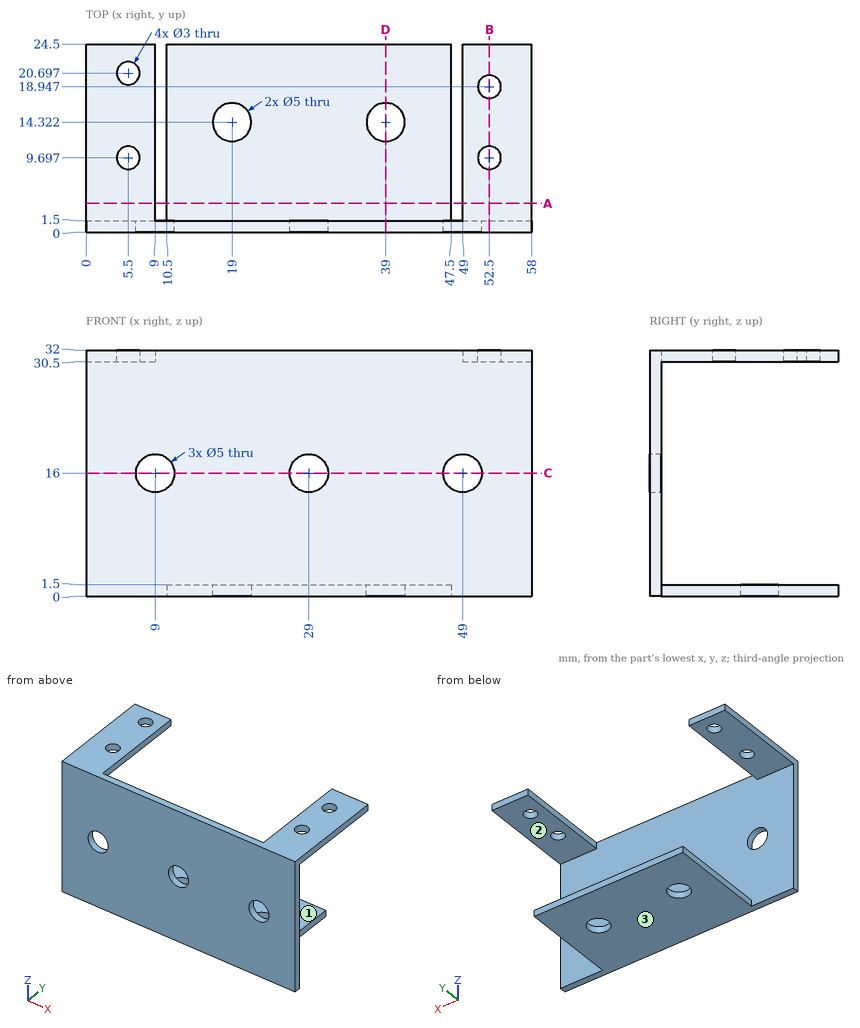
Job drawing, mm, ordinate dimensions from the low corner. One solid piece. A direction names the side the tool comes from. Coordinates: 2 decimals unless noted, no trailing zeros. Write each loop counter-clockwise with the first axis right and the second up, starting at its lowest first coordinate (ties: lowest second). Pieces come first, ordered by that corner, then holes.
Item 1: Which spindle directions (+Z, -Z, +X, -X, +Y, -Y) get a long thin tool onto all of the face, cutting with end or side? Do the marked faces 1, 2 and 3. Say none if no direction does.
Item 2: Slice it at B-B (x = 52.5). Write the cut outline in (y, z).
Item 3: Slice it at D-D (x = 39). Write the cut outline in (y, z).
Item 4: Slice it at C-C (z = 16). Write the cut outline in (x, y).
Item 5: Pin check, flat tips, straight feed: pin 1 (0.8 mm diameter, centred on y = 10.5, z = 0.5, fed in from +X); pin 2 (1.2 mm diameter, centred on y = 16, z = 0.5, fed in from -X); pin 3 (5 mm diameter, centred on x = 5.5, y = 9.7, fed in from -Z); pin 4 (4.5 mm diameter, centred on x = 29, z = 16, fed in from -Y). Stop position of each tip, or through.
Item 6: Probe line 1 (X direction, y = 0.85, z = 16); line 2 (Y direction, x = 52.5, z = 31.2); line 3 (Y direction, x = 5.5, z = 30.95). List the from-to ranges inside material, lowest first.
Item 7: Slice it at A-A (y = 3.75). Write the cut outline in (x, z).
Results found:
1. face 1: +Z, +X, -X, +Y
1. face 2: -Z, +X, -X, +Y
1. face 3: -Z, +X, -X, +Y, -Y
2. outline: (0, 0) - (1.5, 0) - (1.5, 30.5) - (8.2, 30.5) - (8.2, 32) - (0, 32) - close; (11.2, 30.5) - (17.45, 30.5) - (17.45, 32) - (11.2, 32) - close; (20.45, 30.5) - (24.5, 30.5) - (24.5, 32) - (20.45, 32) - close
3. outline: (0, 0) - (11.82, 0) - (11.82, 1.5) - (1.5, 1.5) - (1.5, 32) - (0, 32) - close; (16.82, 0) - (24.5, 0) - (24.5, 1.5) - (16.82, 1.5) - close
4. outline: (0, 0) - (6.5, 0) - (6.5, 1.5) - (0, 1.5) - close; (11.5, 0) - (26.5, 0) - (26.5, 1.5) - (11.5, 1.5) - close; (31.5, 0) - (46.5, 0) - (46.5, 1.5) - (31.5, 1.5) - close; (51.5, 0) - (58, 0) - (58, 1.5) - (51.5, 1.5) - close
5. pin 1: stops at x = 47.5
5. pin 2: stops at x = 10.5
5. pin 3: stops at z = 30.5
5. pin 4: passes through
6. line 1: x = 0 to 6.5, 11.5 to 26.5, 31.5 to 46.5, 51.5 to 58
6. line 2: y = 0 to 8.2, 11.2 to 17.45, 20.45 to 24.5
6. line 3: y = 0 to 8.2, 11.2 to 19.2, 22.2 to 24.5
7. outline: (0, 30.5) - (9, 30.5) - (9, 32) - (0, 32) - close; (10.5, 0) - (47.5, 0) - (47.5, 1.5) - (10.5, 1.5) - close; (49, 30.5) - (58, 30.5) - (58, 32) - (49, 32) - close
